For this review, take the finished solid that the model builds, in its own axes (mm). Round coordinates to 2 decimals unless told otherwise and drop trailing zeros. Write each loop counter-clockwise with the first axis right and the second up, starting at its lowest first coordinate (ties: lowest second). Pieces come first, ordered by that corner, then holes. Notation, with made-up numbers: (34.5, 81) - (53.5, 81) arc R17 cw to (53.5, 96) - close; hole circle Ø5 at (3, 9). An arc over 180 degrees is marked (long way). One line per item, written item: value. Start each with the question number.
Q1. Add section A-A on x = -2.54. Write out the cut boundary in (y, z).
Q2. Add section B-B on z = -99.06. Write out the cut boundary in (x, y), and give its area (3 significant figures).
Q3. Add section D-D on x = -99.06. Write out the cut boundary in (y, z).
Q4. Clearance check with flat-ended pins moving along their axes: pin 1 Ø0.8 at (x, y) = (-102.5, 1) entering from -Z; pin 2 Ø5 at (x, z) = (-99.06, -79.248) entering from +Y; pin 3 Ø0.8 at (y, z) = (0.5, -92) entering from -X. State where each tip first meets the part, or that it passes through.
Q5. For probe 1 along Z at (x, y) = (-2.54, 0.8); probe 2 along Z at (x, y) = (-99.06, 1.2); probe 3 along X at (y, z) = (1, -99.06), list the stretches that pass through material, from the lowest coordinate up.
Q6. Add section C-C on y = 0.7. Write out the cut boundary in (x, z), and give its area (3 significant figures).
Autodesk Inventor part; units mm, degrees
ref_plane "YZ Plane" through (0, 0, 0) normal (1, 0, 0) x (0, 1, 0)
ref_plane "XZ Plane" through (0, 0, 0) normal (0, 1, 0) x (-1, 0, 0)
ref_plane "XY Plane" through (0, 0, 0) normal (0, 0, 1) x (1, 0, 0)
sketch "Sketch1" plane through (0, 0, 0) normal (0, 1, 0) x (-1, 0, 0)
  line L0 (0, 0) -> (104.14, 0)
  line L1 (104.14, 0) -> (104.14, -104.14)
  line L2 (104.14, -104.14) -> (0, -104.14)
  line L3 (0, -104.14) -> (0, 0)
  dimension "d0" = 104.14
  dimension "d1" = 104.14
extrude "Extrusion1" add sketch "Sketch1" along normal blind 1.5748
hole "Hole1" at (-2.54, 1.5748, -5.08) direction (0, -1, 0) diameter 3.2766 depth 25.4
hole "Hole2" at (-2.54, 1.5748, -99.06) direction (0, -1, 0) diameter 3.2766 depth 25.4
sketch "Sketch3" plane through (0, 1.5748, 0) normal (0, 1, 0) x (1, 0, 0)
  line L0 (0, 104.14) -> (-104.14, 104.14)
  line L1 (-104.14, 104.14) -> (-97.5106, 104.14)
  line L2 (-97.5106, 104.14) -> (-97.5106, 84.328)
  line L3 (-97.5106, 84.328) -> (-104.14, 84.328)
  line L4 (-104.14, 84.328) -> (-104.14, 104.14)
  line L5 (-104.14, 0) -> (0, 0)
  dimension "d46" = 6.6294
  dimension "d47" = 84.328
extrude "Extrusion3" cut sketch "Sketch3" against normal blind 25.4
hole "Hole5" at (-99.06, 1.5748, -79.248) direction (0, -1, 0) diameter 3.2766 depth 25.4
hole "Hole6" at (-99.06, 1.5748, -43.434) direction (0, -1, 0) diameter 3.2766 depth 25.4
properties part number "PCB"
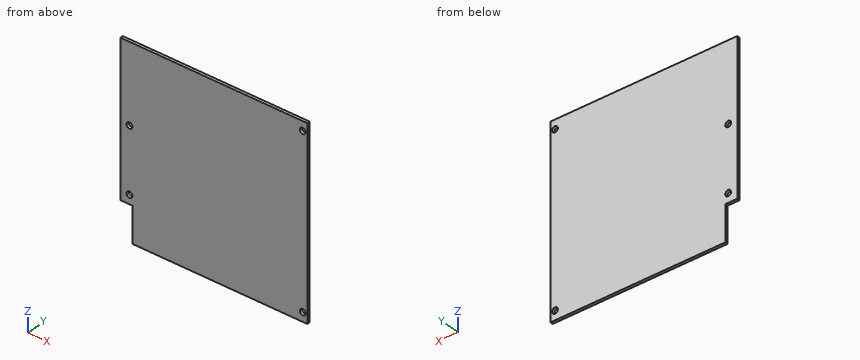
Result set:
1. outline: (0, -104.14) - (1.57, -104.14) - (1.57, -100.7) - (0, -100.7) - close; (0, -97.42) - (1.57, -97.42) - (1.57, -6.72) - (0, -6.72) - close; (0, -3.44) - (1.57, -3.44) - (1.57, 0) - (0, 0) - close
2. outline: (-97.51, 0) - (-4.18, 0) - (-4.18, 1.57) - (-97.51, 1.57) - close; (-0.9, 0) - (0, 0) - (0, 1.57) - (-0.9, 1.57) - close
2. area: 148 mm^2
3. outline: (0, -84.33) - (1.57, -84.33) - (1.57, -80.89) - (0, -80.89) - close; (0, -77.61) - (1.57, -77.61) - (1.57, -45.07) - (0, -45.07) - close; (0, -41.8) - (1.57, -41.8) - (1.57, 0) - (0, 0) - close
4. pin 1: stops at z = -84.33
4. pin 2: stops at y = 1.57
4. pin 3: stops at x = -97.51
5. probe 1: z = -104.14 to -100.7, -97.42 to -6.72, -3.44 to 0
5. probe 2: z = -84.33 to -80.89, -77.61 to -45.07, -41.8 to 0
5. probe 3: x = -97.51 to -4.18, -0.9 to 0
6. outline: (-104.14, -84.33) - (-97.51, -84.33) - (-97.51, -104.14) - (0, -104.14) - (0, 0) - (-104.14, 0) - close; hole circle Ø3.28 at (-99.06, -79.25); hole circle Ø3.28 at (-99.06, -43.43); hole circle Ø3.28 at (-2.54, -99.06); hole circle Ø3.28 at (-2.54, -5.08)
6. area: 10,700 mm^2
